Design review of the part built by this model. Coordinates are the model's own, in mm. A direction names the side the tool comes from. Coordinates: 2 decimals unless noted, no trailing zeros. Order: outer loops, then holes, each group sorted by start corner. A loop starts at its lowest first (then second) coordinate and runs counter-clockwise, first axis right, second up. Notation, with made-up numbers: M 4,-35.75 L 10,-35.75 A19 cw 10,-30.75 Z; hole C 77.5,37 d8. An arc over 180 degrees is marked long. Answer in a Markdown table with one row per item.
from build123d import *

# Parameters (mm, degrees)
BOSS_EXTRUDE1_DEPTH                              = 38.1
BOSS_EXTRUDE1_DRAFT                              = 8
CUT_EXTRUDE1_DEPTH                               = 19.05
CUT_EXTRUDE1_DRAFT                               = -5
CUT_EXTRUDE1_PROFILE_2_DEPTH                     = 19.05
CUT_EXTRUDE1_PROFILE_2_DRAFT                     = -5
CUT_EXTRUDE2_DEPTH                               = 25.4
CUT_EXTRUDE2_DRAFT                               = -8
CBORE_FOR_3_8_SOCKET_HEAD_CAP_SCREW1_D           = 10.3124
CBORE_FOR_3_8_SOCKET_HEAD_CAP_SCREW1_CBORE_D     = 15.875
CBORE_FOR_3_8_SOCKET_HEAD_CAP_SCREW1_CBORE_DEPTH = 9.525


with BuildPart() as part:
    # Sketch1 → Boss-Extrude1 (with draft: the straight prism first)
    with BuildSketch(Plane(origin=(0, 0, 0), x_dir=(0, 1, 0), z_dir=(0, 0, 1))):
        with BuildLine():
            ThreePointArc((-72.39, 57.15), (-79.574204897, 54.174204897), (-82.55, 46.99))
            Line((-82.55, 46.99), (-82.55, -46.99))
            ThreePointArc((-82.55, -46.99), (-79.574204897, -54.174204897), (-72.39, -57.15))
            Line((-72.39, -57.15), (72.39, -57.15))
            ThreePointArc((72.39, -57.15), (79.574204897, -54.174204897), (82.55, -46.99))
            Line((82.55, -46.99), (82.55, 46.99))
            ThreePointArc((82.55, 46.99), (79.574204897, 54.174204897), (72.39, 57.15))
            Line((72.39, 57.15), (-72.39, 57.15))
        make_face()
    extrude(amount=-BOSS_EXTRUDE1_DEPTH)
    # Boss-Extrude1: the draft: its side faces are tilted about the plane it starts from
    boss_extrude1_sides = [part.faces().sort_by_distance(p)[0] for p in [
        (-57.15, 0, -19.05),
        (-54.174204897, -79.574204897, -19.05),
        (0, -82.55, -19.05),
        (54.174204897, -79.574204897, -19.05),
        (57.15, 0, -19.05),
        (54.174204897, 79.574204897, -19.05),
        (0, 82.55, -19.05),
        (-54.174204897, 79.574204897, -19.05),
    ]]
    draft(boss_extrude1_sides, Plane(origin=(0, 0, 0), x_dir=(0, 1, 0), z_dir=(0, 0, 1)), BOSS_EXTRUDE1_DRAFT)


with BuildPart() as cut_extrude1_tool:
    # Sketch4 → Cut-Extrude1 (with draft: the straight prism first)
    with BuildSketch(Plane(origin=(0, 0, 0), x_dir=(0, 1, 0), z_dir=(0, 0, 1))):
        with BuildLine():
            Line((25.4, 19.05), (50.8, 19.05))
            ThreePointArc((50.8, 19.05), (55.290128061, 20.909871939), (57.15, 25.4))
            Line((57.15, 25.4), (57.15, 38.1))
            ThreePointArc((57.15, 38.1), (55.290128061, 42.590128061), (50.8, 44.45))
            Line((50.8, 44.45), (25.4, 44.45))
            ThreePointArc((25.4, 44.45), (20.909871939, 42.590128061), (19.05, 38.1))
            Line((19.05, 38.1), (19.05, 25.4))
            ThreePointArc((19.05, 25.4), (20.909871939, 20.909871939), (25.4, 19.05))
        make_face()
    extrude(amount=-CUT_EXTRUDE1_DEPTH)
    # Cut-Extrude1: the draft: its side faces are tilted about the plane it starts from
    cut_extrude1_sides = [cut_extrude1_tool.faces().sort_by_distance(p)[0] for p in [
        (-20.909871939, 20.909871939, -9.525),
        (-19.05, 38.1, -9.525),
        (-20.909871939, 55.290128061, -9.525),
        (-31.75, 57.15, -9.525),
        (-42.590128061, 55.290128061, -9.525),
        (-44.45, 38.1, -9.525),
        (-42.590128061, 20.909871939, -9.525),
        (-31.75, 19.05, -9.525),
    ]]
    draft(cut_extrude1_sides, Plane(origin=(0, 0, 0), x_dir=(0, 1, 0), z_dir=(0, 0, 1)), CUT_EXTRUDE1_DRAFT)


with BuildPart() as part_1:
    add(part.part)

    # Cut-Extrude1: cut by cut_extrude1_tool
    add(cut_extrude1_tool.part, mode=Mode.SUBTRACT)


with BuildPart() as cut_extrude1_profile_2_tool:
    # Sketch4 → Cut-Extrude1 profile 2 (with draft: the straight prism first)
    with BuildSketch(Plane(origin=(0, 0, 0), x_dir=(0, 1, 0), z_dir=(0, 0, 1))):
        with BuildLine():
            Line((6.35, -12.7), (6.35, -38.1))
            ThreePointArc((6.35, -38.1), (8.209871939, -42.590128061), (12.7, -44.45))
            Line((12.7, -44.45), (63.5, -44.45))
            ThreePointArc((63.5, -44.45), (67.990128061, -42.590128061), (69.85, -38.1))
            Line((69.85, -38.1), (69.85, -12.7))
            ThreePointArc((69.85, -12.7), (67.990128061, -8.209871939), (63.5, -6.35))
            Line((63.5, -6.35), (12.7, -6.35))
            ThreePointArc((12.7, -6.35), (8.209871939, -8.209871939), (6.35, -12.7))
        make_face()
    extrude(amount=-CUT_EXTRUDE1_PROFILE_2_DEPTH)
    # Cut-Extrude1 profile 2: the draft: its side faces are tilted about the plane it starts from
    cut_extrude1_profile_2_sides = [cut_extrude1_profile_2_tool.faces().sort_by_distance(p)[0] for p in [
        (25.4, 6.35, -9.525),
        (42.590128061, 8.209871939, -9.525),
        (44.45, 38.1, -9.525),
        (42.590128061, 67.990128061, -9.525),
        (25.4, 69.85, -9.525),
        (8.209871939, 67.990128061, -9.525),
        (6.35, 38.1, -9.525),
        (8.209871939, 8.209871939, -9.525),
    ]]
    draft(cut_extrude1_profile_2_sides, Plane(origin=(0, 0, 0), x_dir=(0, 1, 0), z_dir=(0, 0, 1)), CUT_EXTRUDE1_PROFILE_2_DRAFT)


with BuildPart() as part_2:
    add(part_1.part)

    # Cut-Extrude1 profile 2: cut by cut_extrude1_profile_2_tool
    add(cut_extrude1_profile_2_tool.part, mode=Mode.SUBTRACT)


with BuildPart() as cut_extrude2_tool:
    # Sketch4<3> → Cut-Extrude2 (with draft: the straight prism first)
    with BuildSketch(Plane(origin=(0, 0, 0), x_dir=(0, 1, 0), z_dir=(0, 0, 1))):
        with BuildLine():
            ThreePointArc((-63.5, 44.45), (-67.990128061, 42.590128061), (-69.85, 38.1))
            Line((-69.85, 38.1), (-69.85, -38.1))
            ThreePointArc((-69.85, -38.1), (-67.990128061, -42.590128061), (-63.5, -44.45))
            Line((-63.5, -44.45), (-25.4, -44.45))
            ThreePointArc((-25.4, -44.45), (-20.909871939, -42.590128061), (-19.05, -38.1))
            Line((-19.05, -38.1), (-19.05, 38.1))
            ThreePointArc((-19.05, 38.1), (-20.909871939, 42.590128061), (-25.4, 44.45))
            Line((-25.4, 44.45), (-63.5, 44.45))
        make_face()
    extrude(amount=-CUT_EXTRUDE2_DEPTH)
    # Cut-Extrude2: the draft: its side faces are tilted about the plane it starts from
    cut_extrude2_sides = [cut_extrude2_tool.faces().sort_by_distance(p)[0] for p in [
        (-42.590128061, -20.909871939, -12.7),
        (-44.45, -44.45, -12.7),
        (-42.590128061, -67.990128061, -12.7),
        (0, -69.85, -12.7),
        (42.590128061, -67.990128061, -12.7),
        (44.45, -44.45, -12.7),
        (42.590128061, -20.909871939, -12.7),
        (0, -19.05, -12.7),
    ]]
    draft(cut_extrude2_sides, Plane(origin=(0, 0, 0), x_dir=(0, 1, 0), z_dir=(0, 0, 1)), CUT_EXTRUDE2_DRAFT)


with BuildPart() as part_3:
    add(part_2.part)

    # Cut-Extrude2: cut by cut_extrude2_tool
    add(cut_extrude2_tool.part, mode=Mode.SUBTRACT)

    # CBORE for 3/8 Socket Head Cap Screw1 (through all)
    with Locations(Plane(origin=(0, 0, 0), x_dir=(0, -1, 0), z_dir=(0, 0, 1))):
        with Locations((0, 0)):
            CounterBoreHole(CBORE_FOR_3_8_SOCKET_HEAD_CAP_SCREW1_D / 2, CBORE_FOR_3_8_SOCKET_HEAD_CAP_SCREW1_CBORE_D / 2, CBORE_FOR_3_8_SOCKET_HEAD_CAP_SCREW1_CBORE_DEPTH)


solid = part_3.part
(1) Add section D-D, the plane x = -35. Give the boundary of the cut face in (y, z), and give its area (3 significant figures).
Return value:
| item | result |
|---|---|
| outline | M -87.9,-38.1 L 87.9,-38.1 L 82.55,0 L 57.15,0 L 55.48,-19.05 L 20.72,-19.05 L 19.05,0 L -19.05,0 L -22.62,-25.4 L -66.28,-25.4 L -69.85,0 L -82.55,0 Z |
| area | 4,600 mm2 |
(2) For line 1 along Y through (x, z) = (11.5, -2); line 2 along X through (y, z) = (40, -5); line 3 along Y through (x, z) = (-38, -17), list the stretches that pass through material, from the lowest coordinate up. Write a range as from..to.
Return value:
| item | result |
|---|---|
| line 1 | y = -82.83..-69.57, -19.33..6.64, 69.56..82.83 |
| line 2 | x = -57.85..-44.01, -19.49..6.79, 44.01..57.85 |
| line 3 | y = -84.94..-67.46, -21.44..20.54, 55.66..84.94 |
(3) Add section C-C, the plane z = -23.5. Give the boundary of the cut face in (x, y).
Return value:
| item | result |
|---|---|
| outline | M -60.45,-72.39 A13.46 ccw -46.99,-85.85 L 46.99,-85.85 A13.46 ccw 60.45,-72.39 L 60.45,72.39 A13.46 ccw 46.99,85.85 L -46.99,85.85 A13.46 ccw -60.45,72.39 Z; hole M -41.15,-63.5 A3.05 ccw -38.1,-66.55 L 38.1,-66.55 A3.05 ccw 41.15,-63.5 L 41.15,-25.4 A3.05 ccw 38.1,-22.35 L -38.1,-22.35 A3.05 ccw -41.15,-25.4 Z; hole C 0,0 d10.31 |
(4) Draft analysis for pull direction Y (two halves, no side actions). For faces 3 (the flat face through (7.17, 38.46, -9.39)), 4 (the conical face through (-55.94, 81.54, -18.78)), 5 (the flat face through (-59.79, 1.01, -18.78)), state which applies: pulls with the +Y half, pulls with the -Y half, needs draft (parallel to the pull), parting line crosses it, or undercut.
Return value:
| item | result |
|---|---|
| face 3 | undercut |
| face 4 | pulls with the +Y half |
| face 5 | needs draft |
(5) For faces 1 (the flat face through (25.22, 7.17, -9.39)), 2 (the flat face through (-14, -1, 0)), list the 3-axis set-ups (+Z, -Z, +X, -X, +Y, -Y) from which the entire face can be reached by the end or side of a thin tool; tool diameter is ignored.
Return value:
| item | result |
|---|---|
| face 1 | +Z |
| face 2 | +Z, +X, -X, +Y, -Y |
(6) Insertion check: pin 1 Ø8 at (y, z) = (-5, -6) entering from +X; pin 2 Ø6 at (x, y) = (0, 0) entering from -Z; pin 3 Ø2 at (x, z) = (-42, -33) entering from +Y; pin 4 Ø5 at (x, y) = (3.5, -1) entering from +Z (3 decimals). Each pin has a flat end and moves straight along its axis. Give the tip position at first contact, or say it passes through.
Return value:
| item | result |
|---|---|
| pin 1 | stops at x = 58.56 |
| pin 2 | passes through |
| pin 3 | stops at y = 87.33 |
| pin 4 | stops at z = -9.525 |
